Work out the finished part from the listing and answer in its coordinate system (mm). Coordinates: 2 decimals unless noted, no trailing zeros. Order: outer loops, then holes, each group sorted by start corner. A loop starts at its lowest first (then second) coordinate and runs counter-clockwise, first axis right, second up. Notation, with made-up numbers: M 43,11.25 L 91,11.25 A24 cw 91,24.25 Z; hole C 65,52.5 d11. An arc over 180 degrees is marked long. Use a Markdown table: item, result.
from build123d import *

# Parameters (mm, degrees)
CROQUIS1_R              = 15
SALIENTE_EXTRUIR1_DEPTH = 170
CROQUIS2_R              = 15
CROQUIS3_R              = 15
SALIENTE_EXTRUIR2_DEPTH = 20


with BuildPart() as part:
    # Croquis1 → Saliente-Extruir1 (new body)
    with BuildSketch(Plane.XY):
        Circle(CROQUIS1_R)
    extrude(amount=SALIENTE_EXTRUIR1_DEPTH)

    # Barrer1: sweep along a curve in space
    with BuildLine() as barrer1_path:
        Line((0, 0, 170), (0, 0, 177.4880174))
        ThreePointArc((0, 0, 177.4880174), (0, 1.310507191, 188.860496902), (0, 5.173331601, 199.636827757))
        Line((0, 5.173331601, 199.636827757), (0, 17.719048286, 225.027928795))
    # Croquis2 → Barrer1 (sweep)
    with BuildSketch(Plane.XY.offset(170)):
        Circle(CROQUIS2_R)
    sweep(path=barrer1_path.line)

    # Croquis3 → Saliente-Extruir2 (add)
    with BuildSketch(Plane(origin=(0, 0, 0), x_dir=(-1, 0, 0), z_dir=(0, 0, -1))):
        Circle(CROQUIS3_R)
    extrude(amount=SALIENTE_EXTRUIR2_DEPTH)


solid = part.part
1. Section B-B on z = 41.5 is taken. Determine the outline of the cut face in (x, y), then the cut area to 3 significant figures.
Answers below:
| item | result |
|---|---|
| outline | C 0,0 d30 |
| area | 707 mm² |
2. Section A-A on x = 0 is taken. Determine the outline of the cut face in (y, z), then the cut area to 3 significant figures.
Answers below:
| item | result |
|---|---|
| outline | M -15,-20 L 15,-20 L 15,177.49 A35 cw 18.62,192.99 L 31.17,218.38 L 4.27,231.67 L -8.27,206.28 A65 ccw -15,177.49 Z |
| area | 7,460 mm² |
3. Section C-C on x = 10.5 is taken. Determine the outline of the cut face in (y, z), then the cut area to 3 significant figures.
Answers below:
| item | result |
|---|---|
| outline | M -10.71,-20 L 10.71,-20 L 10.71,177.49 A39.29 cw 14.78,194.89 L 27.32,220.28 L 8.12,229.77 L -4.43,204.38 A60.71 ccw -10.71,177.49 Z |
| area | 5,330 mm² |
4. Flat-ended cylindrical pins translate along their axes: P1, Ø8, axis at x = -5, z = 7.5, coming from the -Y side; P2, Ø8, axis at x = 10, z = 132.5, coming from the -Y side; P3, Ø1.5, axis at x = -11.5, y = 20.5, coming from the +Z side. Find the tip coordinate at first contact, or state that the pin passes through.
Answers below:
| item | result |
|---|---|
| P1 | y = -14.97 |
| P2 | y = -13.75 |
| P3 | z = 224.02 |
5. Find the intervals of material crossed by probe 1 along Y at (x, z) = (0, 19); probe 2 along Y at (x, z) = (7, 63.5); probe 3 along X at (y, z) = (-7.5, 160), in increasing order.
Answers below:
| item | result |
|---|---|
| probe 1 | -15 to 15 |
| probe 2 | -13.27 to 13.27 |
| probe 3 | -12.99 to 12.99 |
